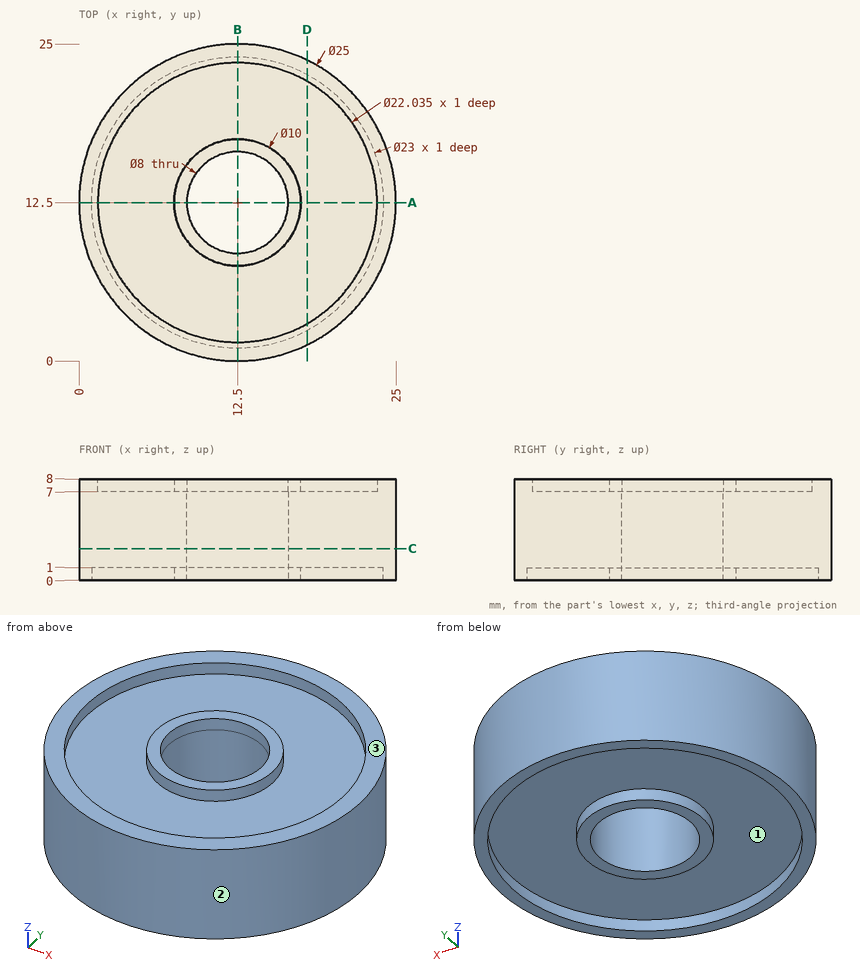
Check sheet for the drawn part. Datum: minimum x, y, z corner. Units: mm. Round coordinates to 2 decimals unless told otherwise and drop trailing zeros. Write each loop counter-clockwise with the first axis right and the second up, starting at its lowest first coordinate (ties: lowest second). Pieces come first, ordered by that corner, then holes. Notation, with made-up numbers: (49.5, 88) - (88.5, 88) arc R16 ccw to (88.5, 115) - close; hole circle Ø10 at (3, 37.5). An arc over 180 degrees is marked (long way). Return JSON: item names as keys, results as strings.
Q1. Scan lines: L1, parallel to Y at x = 12.5, z = 0.5; L2, parallel to X at y = 12.25, z = 6.5; L3, parallel to Y at x = 12.5, z = 2.5. Record each from-to range of solid material in increasing order. Write a range as from..to.
Returned:
{"L1": "y = 0..1, 7.5..8.5, 16.5..17.5, 24..25", "L2": "x = 0..8.51, 16.49..25", "L3": "y = 0..8.5, 16.5..25"}
Q2. Draft check along Y on the marked faces 1, 2 and 3. Enter one of: released by +Y, released by -Y, zero draft, split by the parting line, or undercut.
Returned:
{"face 1": "undercut", "face 2": "split by the parting line", "face 3": "zero draft"}
Q3. Depth check by flat-ended pin: P1, Ø4, axis at y = 6.5, z = 1, coming from the -X side; P2, Ø11.5, axis at x = 16, y = 17.5, coming from the -Z side; P3, Ø1.5, axis at y = 14, z = 1, coming from the +X side; P4, Ø3, axis at x = 4, y = 12.5, coming from the +Z side. Enter the tip coordinate at first touch or a pass-through.
Returned:
{"P1": "stops at x = 0.66", "P2": "stops at z = 0", "P3": "stops at x = 24.98", "P4": "stops at z = 7"}
Q4. Cross-section at D-D (x = 18). Record the boundary of the cut face in (y, z) (1 decimal), then the cut area to 3 significant figures.
Returned:
{"outline": "(1.3, 0) - (2.4, 0) - (2.4, 1) - (22.6, 1) - (22.6, 0) - (23.7, 0) - (23.7, 8) - (22, 8) - (22, 7) - (3, 7) - (3, 8) - (1.3, 8) - close", "area": "140 mm²"}
Q5. Cross-section at C-C (z = 2.5). Record the boundary of the cut face in (x, y).
Returned:
{"outline": "circle Ø25 at (12.5, 12.5); hole circle Ø8 at (12.5, 12.5)"}
Q6. Cross-section at A-A (y = 12.5). Record the boundary of the cut face in (x, z), then the cut area to 3 significant figures.
Returned:
{"outline": "(0, 0) - (1, 0) - (1, 1) - (7.5, 1) - (7.5, 0) - (8.5, 0) - (8.5, 8) - (7.5, 8) - (7.5, 7) - (1.48, 7) - (1.48, 8) - (0, 8) - close; (16.5, 0) - (17.5, 0) - (17.5, 1) - (24, 1) - (24, 0) - (25, 0) - (25, 8) - (23.52, 8) - (23.52, 7) - (17.5, 7) - (17.5, 8) - (16.5, 8) - close", "area": "111 mm²"}
